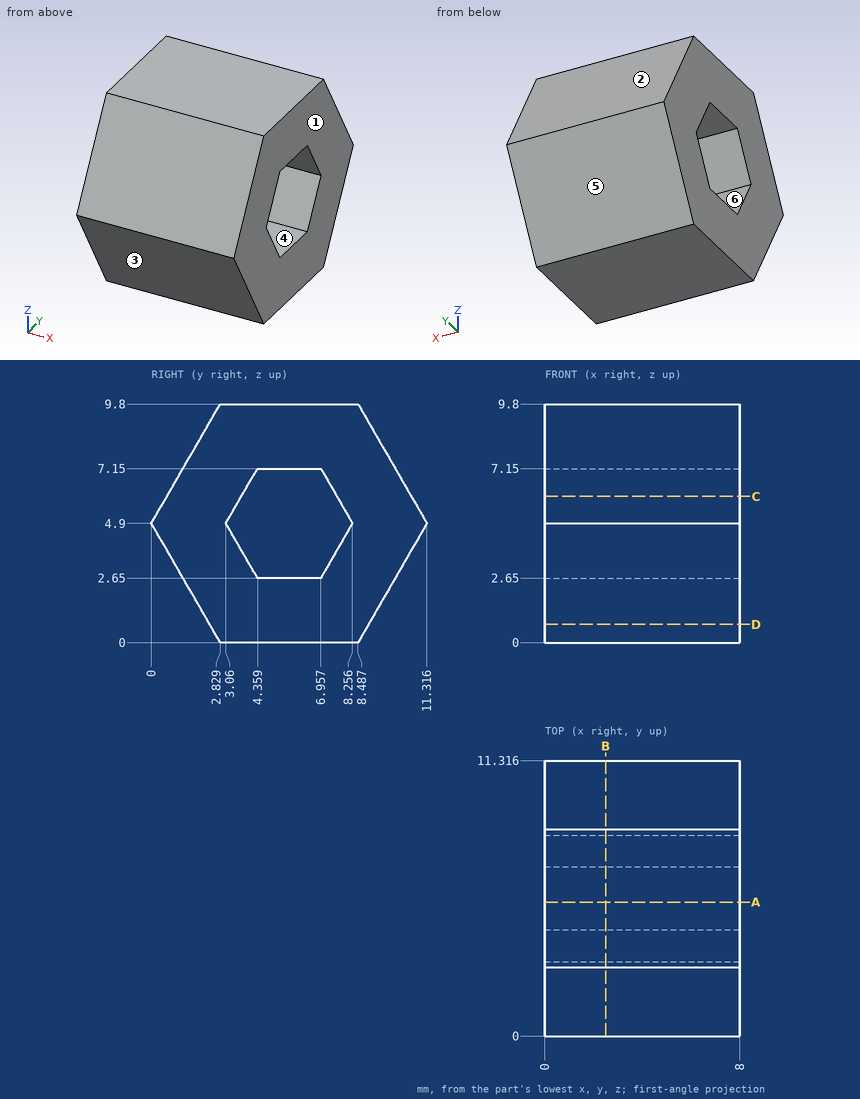
Check sheet for the drawn part. Datum: minimum x, y, z corner. Units: mm. A direction names the side the tool comes from. Coordinates: 2 decimals unless noted, no trailing zeros. Loops run counter-clockwise (first coordinate to the right, second up) from the corner with the lowest first, then second, coordinate; pieces in that order, holes last. Notation, with made-up numbers: M 18,41 L 63,41 A13 cw 63,56 Z; hole C 57,-30 d7. An arc over 180 degrees is marked long. Answer as a JSON object with one key per item and string values.
1. Depth check by flat-ended pin: P1, Ø1.5, axis at x = 5.5, z = 8, coming from the +Y side; P2, Ø3, axis at x = 4.5, z = 1.5, coming from the -Y side; P3, Ø2, axis at x = 6.5, z = 6, coming from the -Y side. Enter the tip coordinate at first touch or a pass-through.
Outcome:
{"P1": "y = 9.96", "P2": "y = 1.1", "P3": "y = 0.06"}
2. Sectioned sample at C-C on z = 6. Record the cut outline in (x, y) (3 decimals).
Outcome:
{"outline": "M 0,0.635 L 8,0.635 L 8,3.695 L 0,3.695 Z; M 0,7.621 L 8,7.621 L 8,10.681 L 0,10.681 Z"}
3. Access from +Z, -Z, +X, -X, +Y, -Y to the whole of each face (thin tool, end or side, straight path). Record for the marked faces 5 and 6.
Outcome:
{"face 5": "-Z, +X, -X, +Y", "face 6": "+X, -X"}
4. Release check for a two-part mould opening along Y. For the marked faces 1, 2, 3 and 4 record: pulls with the +Y half, pulls with the -Y half, needs draft (parallel to the pull), parting line crosses it, or undercut.
Outcome:
{"face 1": "needs draft", "face 2": "pulls with the +Y half", "face 3": "pulls with the -Y half", "face 4": "undercut"}
5. Sectioned sample at D-D on z = 0.75. Record the cut outline in (x, y), and give its area (3 significant figures).
Outcome:
{"outline": "M 0,2.4 L 8,2.4 L 8,8.92 L 0,8.92 Z", "area": "52.2 mm²"}
6. Scan lines: L1, parallel to Z at x = 6, y = 6.5; L2, parallel to Y at x = 1.5, z = 4; L3, parallel to Y at x = 3.5, z = 5.75 (1 decimal). Record each from-to range of solid material in increasing order. Write a range as from..to.
Outcome:
{"L1": "0..2.65, 7.15..9.8", "L2": "0.52..3.58, 7.74..10.8", "L3": "0.5..3.6, 7.8..10.8"}
7. Sectioned sample at B-B on x = 2.5. Record the cut outline in (y, z), and give its area (3 significant figures).
Outcome:
{"outline": "M 0,4.9 L 2.83,0 L 8.49,0 L 11.32,4.9 L 8.49,9.8 L 2.83,9.8 Z; hole M 3.06,4.9 L 4.36,2.65 L 6.96,2.65 L 8.26,4.9 L 6.96,7.15 L 4.36,7.15 Z", "area": "65.6 mm²"}
8. Sectioned sample at A-A on y = 5.5. Record the cut outline in (x, z), and give its area (3 significant figures).
Outcome:
{"outline": "M 0,0 L 8,0 L 8,2.65 L 0,2.65 Z; M 0,7.15 L 8,7.15 L 8,9.8 L 0,9.8 Z", "area": "42.4 mm²"}
